```python
from build123d import *

# Parameters (mm, degrees)
F0_R     = 6.35
F0_R_2   = 4.826
F1_DEPTH = 17.78
F2_DEPTH = 3.96875
F3_R     = 3.3655
F4_DEPTH = 11.9126
F8_DEPTH = 11.0998


with BuildPart() as f1:
    # F0 (on Top) → F1 (new body)
    with BuildSketch(Plane.XY):
        Circle(F0_R)
        Circle(F0_R_2, mode=Mode.SUBTRACT)
        Circle(F0_R_2)
    extrude(amount=-F1_DEPTH)

    # F0 (on Top) → F2 (cut)
    with BuildSketch(Plane.XY):
        Circle(F0_R_2)
    extrude(amount=-F2_DEPTH, mode=Mode.SUBTRACT)

    # F3 (on face) → F4 (cut)
    with BuildSketch(Plane.XY.offset(-3.96875)):
        Circle(F3_R)
    extrude(amount=-F4_DEPTH, mode=Mode.SUBTRACT)

    # F5 (on Front) → F6 (revolve, cut)
    with BuildSketch(Plane.XZ):
        with BuildLine():
            Line((-6.35, -4.0450559158), (-6.35, -17.78))
            Line((-6.35, -17.78), (-4.699, -17.78))
            Line((-4.699, -17.78), (-4.699, -15.88135))
            add(Edge.make_bspline(
                [(-6.35, -2.0225279579), (-6.35, -6.1770705744), (-5.3292767375, -5.3773556727), (-4.699, -11.7937795575), (-4.699, -15.88135)],
                knots=[0, 0, 0, 0, 0.4207974833, 1, 1, 1, 1], degree=3))
            Line((-6.35, -2.0225279579), (-6.35, -4.0450559158))
        make_face()
        Polygon((-4.699, -17.78), (-6.35, -17.78), (-6.35, -4.0450559158), (-6.35, -2.0225279579), (-8.8478010148, -2.0225279579), (-8.8478010148, -19.1934037815), (-4.699, -19.1934037815), align=None)
    revolve(axis=Axis((0, 0, -1.0444802465), (0, 0, -1)), mode=Mode.SUBTRACT)

    # F7 (on face) → F8 (join)
    with BuildSketch(Plane(origin=(0, 0, -17.78), x_dir=(1, 0, 0), z_dir=(0, 0, -1))):
        with BuildLine():
            ThreePointArc((2.4113470969, -4.0331137076), (3.9334862522, -3.9334862522), (4.0331137076, -2.4113470969))
            ThreePointArc((4.0331137076, -2.4113470969), (3.3226947648, -3.3226947648), (2.4113470969, -4.0331137076))
        make_face()
        with BuildLine():
            ThreePointArc((-1.1467621679, -4.5569219359), (0, -5.5627896053), (1.1467621679, -4.5569219359))
            ThreePointArc((1.1467621679, -4.5569219359), (0, -4.699), (-1.1467621679, -4.5569219359))
        make_face()
        with BuildLine():
            ThreePointArc((-4.0331137076, -2.4113470969), (-3.9334862522, -3.9334862522), (-2.4113470969, -4.0331137076))
            ThreePointArc((-2.4113470969, -4.0331137076), (-3.3226947648, -3.3226947648), (-4.0331137076, -2.4113470969))
        make_face()
        with BuildLine():
            ThreePointArc((-4.5569219359, -1.1467621679), (-4.699, 0), (-4.5569219359, 1.1467621679))
            ThreePointArc((-4.5569219359, 1.1467621679), (-5.5627896053, 0), (-4.5569219359, -1.1467621679))
        make_face()
        with BuildLine():
            ThreePointArc((-4.0331137076, 2.4113470969), (-3.3226947648, 3.3226947648), (-2.4113470969, 4.0331137076))
            ThreePointArc((-2.4113470969, 4.0331137076), (-3.9334862522, 3.9334862522), (-4.0331137076, 2.4113470969))
        make_face()
        with BuildLine():
            ThreePointArc((-1.1467621679, 4.5569219359), (0, 4.699), (1.1467621679, 4.5569219359))
            ThreePointArc((1.1467621679, 4.5569219359), (0, 5.5627896053), (-1.1467621679, 4.5569219359))
        make_face()
        with BuildLine():
            ThreePointArc((2.4113470969, 4.0331137076), (3.3226947648, 3.3226947648), (4.0331137076, 2.4113470969))
            ThreePointArc((4.0331137076, 2.4113470969), (3.9334862522, 3.9334862522), (2.4113470969, 4.0331137076))
        make_face()
        with BuildLine():
            ThreePointArc((4.5569219359, 1.1467621679), (4.6633452144, 0.5777650141), (4.699, 0))
            ThreePointArc((4.699, 0), (4.6633452144, -0.5777650141), (4.5569219359, -1.1467621679))
            ThreePointArc((4.5569219359, -1.1467621679), (5.5627896053, 0), (4.5569219359, 1.1467621679))
        make_face()
    extrude(amount=-F8_DEPTH)


solid = f1.part
```
Build history of the part. All positions in model axes, mm. A direction names the side the tool comes from. Round coordinates to 2 decimals unless told otherwise and drop trailing zeros.
1) Drill centre lines: probe 1 along Y at (x, z) = (0, -8.25); probe 2 along Y at (x, z) = (0, -2.3); probe 3 along Z at (x, y) = (3, 2.75). Where is each one in solid material? Low to high.
2) Pin check, flat tips, straight feed: pin 1 (4 mm diameter, centred on x = -4, z = -4.5, fed in from +Y); pin 2 (4 mm diameter, centred on x = -5, z = -12.5, fed in from +Y); pin 3 (2 mm diameter, centred on y = 3.5, z = -14, fed in from -X). Stop position of each tip, or through.
3) 3-axis set-ups, long thin cutter, end or side, ignore diameter. For faces 1 (the cylindrical face through (-3.917, -3.95, -12.354)), 2 (the cylindrical face through (0.023, -5.563, -12.354)), 3 (the flat face through (0, 0, -15.881)): which of +Z, -Z, +X, -X, +Y, -Y reach the whole face in a straight line?
4) Mould opens along X. For faces 4 (the cylindrical face through (4.338, 1.807, -16.817)), 5 (the cylindrical face through (-3.95, 3.917, -12.354)), 6 (the flat face through (0, 0, -17.78)), 7 (the cylindrical face through (1.807, -4.338, -16.817)) say: +X half, -X half, draft (parallel to the pull), parting line (faces both ways), or undercut.
Ans:
1. probe 1: y = -5.56 to -3.37, 3.37 to 5.56
1. probe 2: y = -6.35 to -4.83, 4.83 to 6.35
1. probe 3: z = -17.78 to -3.97
2. pin 1: stops at y = 5.96
2. pin 2: stops at y = 4.27
2. pin 3: stops at x = -4.27
3. face 1: -Z
3. face 2: -Z, -Y
3. face 3: +Z
4. face 4: +X half
4. face 5: undercut
4. face 6: draft
4. face 7: undercut
